Geometry check sheet. Reference: the model listing, model coordinates, mm. Face numbers are marked on the shaded views. A direction names the side the tool comes from. Round coordinates to 2 decimals unless told otherwise and drop trailing zeros. Loops run counter-clockwise (first coordinate to the right, second up) from the corner with the lowest first, then second, coordinate; pieces in that order, holes last. Notation, with made-up numbers: M 26.5,76 L 36.5,76 A18 ccw 36.5,95 Z; hole C 37.25,65.25 d4. An arc over 180 degrees is marked long. Use one line per item in the form item = value. Start each with the question number.
1. Draft check along X on the marked faces 1, 2 and 3. Enter one of: pulls with the +X half, pulls with the -X half, needs draft (parallel to the pull), parting line crosses it, or undercut.
2. Cross-section at C-C (y = 0). State how many separate pieces and enclosed holes the cut face has, then the cut area to 3 significant figures.
3. Cross-section at D-D (x = -3.5). Record the boundary of the cut face in (y, z).
4. Cross-section at B-B (z = 23.5). Record the boundary of the cut face in (x, y).
5. Material ranges on line 1 (X direction, y = 4, z = 16.5); line 2 (Y direction, x = 0, z = 19.75); line 3 (X direction, y = -1.5, z = 20.5), recorded low to high.
6. Go/stop test with flat-tipped pins: pin 1 (2 mm diameter, centred on x = -11.5, z = 8, fed in from +Y); pin 2 (5.5 mm diameter, centred on x = 21, z = 9, fed in from +Y); pin 3 (5 mm diameter, centred on x = 19, z = 18.5, fed in from +Y). Record where each tip stops, or that it passes through.
7. Set-up check for the marked faces 4, 5 and 6: record each of +Z, -Z, +X, -X, +Y, -Y from which the full face is reachable in a straight line by a thin tool's end or side.
8. Cross-section at A-A (x = 48). Record the boundary of the cut face in (y, z), then the cut area to 3 significant figures.
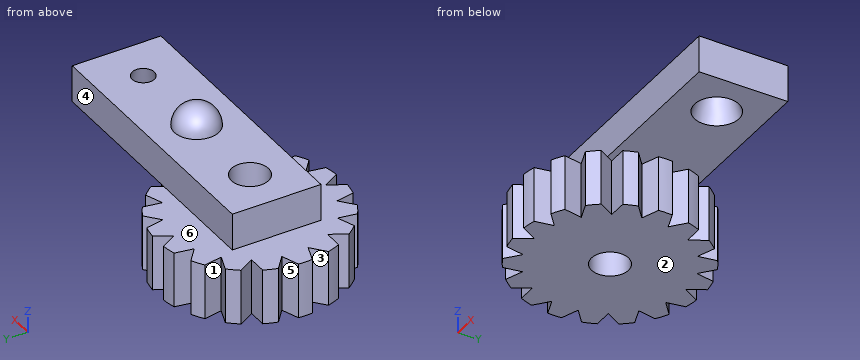
Autodesk Inventor part; units mm, degrees
ref_plane "YZ Plane" through (0, 0, 0) normal (1, 0, 0) x (0, 1, 0)
ref_plane "XZ Plane" through (0, 0, 0) normal (0, 1, 0) x (-1, 0, 0)
ref_plane "XY Plane" through (0, 0, 0) normal (0, 0, 1) x (1, 0, 0)
sketch "Sketch1" plane through (0, 0, 0) normal (0, 0, 1) x (1, 0, 0)
  circle A0 centre (0, 0) radius 25
  circle A1 centre (0, 0) radius 5
  dimension "d0" = 50
  dimension "d1" = 10
extrude "Extrusion1" add sketch "Sketch1" along normal blind 15
sketch "Sketch2" plane through (0, 0, 15) normal (0, 0, 1) x (1, 0, 0)
  circle A0 centre (0, 0) radius 25
  line L0 (0, 25) -> (5, 25) construction
  line L1 (0, 20) -> (6.1776, 20) construction
  line L2 (-2.7962, 24.8431) -> (2.2038, 24.8431) construction
  line L3 (0, 20.5446) -> (2.5, 24.8747)
  line L4 (0, 20.5446) -> (5, 20.5446) construction
  circle A1 centre (0, 0) radius 25
  line L5 (0, 20.5446) -> (0, 24.8431) construction
  line L6 (0, 20.5446) -> (-2.5, 24.8747)
  arc A2 (2.5, 24.8747) -> (-2.5, 24.8747) centre (0, 0) ccw
  dimension "d32" = 5
  dimension "d33" = 60
extrude "Extrusion2" cut sketch "Sketch2" against normal through all contours L3 L6 A0 picked at (1.1115, 23.4685)
pattern_circular "Circular Pattern1" count 18 over 360 about axis through (0, 0, -10) along (0, 0, 1) of "Extrusion2"
sketch "Sketch3" plane through (0, 0, 15) normal (0, 0, 1) x (1, 0, 0)
  line L0 (-12, 12) -> (60, 12)
  line L1 (60, 12) -> (60, -12)
  line L2 (60, -12) -> (-12, -12)
  line L3 (-12, -12) -> (-12, 12)
  circle A0 centre (0, 0) radius 5
  point P0 (-12, 0)
  dimension "d13" = 12
  dimension "d14" = 12
  dimension "d15" = 60
extrude "Extrusion4" add sketch "Sketch3" along normal blind 10
sketch "Sketch4" plane through (0, 0, 15) normal (0, 0, -1) x (-1, 0, 0)
  circle A0 centre (-48, 0) radius 6
  line L0 (-60, 12) -> (-60, -12) construction
  point P0 (0, 0)
  dimension "d20" = 12
  dimension "d21" = 12
sketch "Sketch5" plane through (0, 0, 25) normal (0, 0, 1) x (1, 0, 0)
  circle A0 centre (48, 0) radius 3
  line L0 (60, -12) -> (60, 12) construction
  point P0 (0, 0)
  point P1 (0, 0)
  dimension "d22" = 6
  dimension "d23" = 12
loft "Loft1" cut profiles "Sketch5", "Sketch4"
sketch "Sketch6" plane through (0, 0, 25) normal (0, 0, 1) x (1, 0, 0)
  arc A0 (24, -6) -> (24, 6) centre (24, 0) ccw
  line L0 (-12, -12) -> (60, -12)
  line L1 (24, -6) -> (24, 6)
  point P0 (0, 0)
  point P1 (24, -12)
  dimension "d28" = 12
revolve "Revolution1" add sketch "Sketch6" angle 360 about axis through (24, -6, 25) along (0, 1, 0)
equation "\"d1\" = 0.2 * d0"
equation "\"d21\" = d20"
equation "\"d22\" = 0.5 * d20"
equation "\"d23\" = d21"
properties part number "Parcial3"
Reported:
q1.face_1 = undercut
q1.face_2 = needs draft
q1.face_3 = pulls with the -X half
q2.separate_pieces = 3
q2.enclosed_holes = 0
q2.area = 1,190 mm²
q3.outline = M -24.75,0 L -3.57,0 L -3.57,25 L -12,25 L -12,15 L -24.75,15 Z; M 3.57,0 L 24.75,0 L 24.75,15 L 12,15 L 12,25 L 3.57,25 Z
q4.outline = M -12,-12 L 60,-12 L 60,12 L -12,12 Z; hole C 0,0 d10; hole C 48,0 d6.9
q5.line_1 = -12 to -3, 3 to 44.15, 51.85 to 60
q5.line_2 = -12 to -5, 5 to 12
q5.line_3 = -12 to -4.77, 4.77 to 43.92, 52.08 to 60
q6.pin_1 = 22.52
q6.pin_2 = 17.09
q6.pin_3 = 12
q7.face_4 = +Z, +X, -X, +Y
q7.face_5 = +Z, -Z, -X
q7.face_6 = +Z, -X
q8.outline = M -12,15 L -6,15 L -3,25 L -12,25 Z; M 3,25 L 6,15 L 12,15 L 12,25 Z
q8.area = 150 mm²
